Build history of the part. All positions in model axes, mm. Coordinates: 2 decimals unless noted, no trailing zeros. Loops run counter-clockwise (first coordinate to the right, second up) from the corner with the lowest first, then second, coordinate; pieces in that order, holes last.
(1) Flat gauge pins, fed straight in: P1, Ø1, axis at x = -3.5, y = 107.5, coming from the +Z side; P2, Ø1.6, axis at x = -3, y = 98, coming from the -Z side. Where does each tip first touch, or does it go through?
(2) Slice it at C-C (y = 71.5). Give the cut face in (x, z).
(3) Wall check: L1, parallel to Y at x = -4.4, z = -57.75; L2, parallel to Y at x = -4.5, z = -55; L3, parallel to Z at x = -3.6, y = 88. Give the ranges that are in metal, low to high.
(4) Slice it at B-B (x = -2.9). Give the cut face in (y, z), and give its area (3 significant figures).
(5) Slice it at D-D (y = 101). Give the cut face in (x, z).
(6) Slice it at A-A (z = -56.25). Give the cut face in (x, y).
from build123d import *

# Parameters (mm, degrees)
SKETCH_R  = 3
PAD_DEPTH = 3.175


with BuildPart() as part:
    # Sketch (on Face26 of Binder) → Pad (new body)
    with BuildSketch(Plane.YZ.offset(-1.8542)):
        with BuildLine():
            ThreePointArc((56.923, -48.25), (48.923, -56.25), (56.923, -64.25))
            Line((56.923, -64.25), (73.177, -64.25))
            ThreePointArc((73.177, -64.25), (76.407291, -63.568826), (79.087485, -61.641304))
            ThreePointArc((79.974058, -61.25), (79.489514, -61.352176), (79.087485, -61.641304))
            Line((79.974058, -61.25), (133.829942, -61.25))
            ThreePointArc((134.716515, -61.641304), (134.314486, -61.352176), (133.829942, -61.25))
            ThreePointArc((134.716515, -61.641304), (148.627, -56.25), (134.716515, -50.858696))
            ThreePointArc((133.829942, -51.25), (134.314486, -51.147824), (134.716515, -50.858696))
            Line((79.974058, -51.25), (133.829942, -51.25))
            ThreePointArc((79.087485, -50.858696), (79.489514, -51.147824), (79.974058, -51.25))
            ThreePointArc((79.087485, -50.858696), (76.407291, -48.931174), (73.177, -48.25))
            Line((56.923, -48.25), (73.177, -48.25))
        make_face()
        with Locations((56.923, -56.25)):
            Circle(SKETCH_R, mode=Mode.SUBTRACT)
        with Locations((73.177, -56.25)):
            Circle(SKETCH_R, mode=Mode.SUBTRACT)
        with Locations((140.627, -56.25)):
            Circle(SKETCH_R, mode=Mode.SUBTRACT)
    extrude(amount=-PAD_DEPTH)


solid = part.part
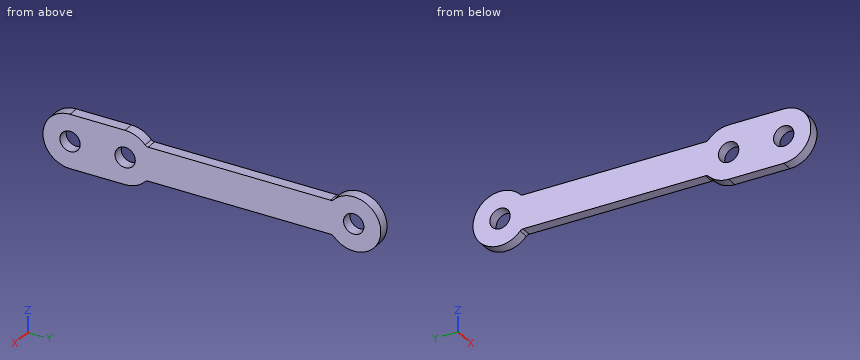
Response values:
1. P1: stops at z = -51.25
1. P2: stops at z = -61.25
2. outline: (-5.03, -64.25) - (-1.85, -64.25) - (-1.85, -58.74) - (-5.03, -58.74) - close; (-5.03, -53.76) - (-1.85, -53.76) - (-1.85, -48.25) - (-5.03, -48.25) - close
3. L1: y = 49.06 to 54.32, 59.52 to 70.58, 75.78 to 138.03, 143.23 to 148.49
3. L2: y = 49.02 to 54.2, 59.65 to 70.45, 75.9 to 137.9, 143.35 to 148.53
3. L3: z = -61.25 to -51.25
4. outline: (56.92, -64.25) - (73.18, -64.25) arc R8 ccw to (79.09, -61.64) arc R1.2 cw to (79.97, -61.25) - (133.83, -61.25) arc R1.2 cw to (134.72, -61.64) arc R8 ccw (long way) to (134.72, -50.86) arc R1.2 cw to (133.83, -51.25) - (79.97, -51.25) arc R1.2 cw to (79.09, -50.86) arc R8 ccw to (73.18, -48.25) - (56.92, -48.25) arc R8 ccw to start; hole circle Ø6 at (56.92, -56.25); hole circle Ø6 at (73.18, -56.25); hole circle Ø6 at (140.63, -56.25)
4. area: 1,100 mm2
5. outline: (-5.03, -61.25) - (-1.85, -61.25) - (-1.85, -51.25) - (-5.03, -51.25) - close
6. outline: (-5.03, 48.92) - (-1.85, 48.92) - (-1.85, 53.92) - (-5.03, 53.92) - close; (-5.03, 59.92) - (-1.85, 59.92) - (-1.85, 70.18) - (-5.03, 70.18) - close; (-5.03, 76.18) - (-1.85, 76.18) - (-1.85, 137.63) - (-5.03, 137.63) - close; (-5.03, 143.63) - (-1.85, 143.63) - (-1.85, 148.63) - (-5.03, 148.63) - close
